Build history of the part. All positions in model axes, mm. A direction names the side the tool comes from. Give positions to 0.01 mm unless a question says otherwise; leave off trailing zeros. Write each loop counter-clockwise with the first axis right and the second up, starting at its lowest first coordinate (ties: lowest second). Pieces come first, ordered by that corner, then holes. Notation, with made-up numbers: (16.5, 54) -> (62.5, 54) arc R18 ccw to (62.5, 67) -> close; hole circle Ø7 at (51.5, -27.5). An arc over 180 degrees is marked (long way). Put each result on its own line as item: value. Start each with the question number.
Item 1: Two-plate mould, pull along Y, no slides. Class faces 1 (the flat face through (8.9, 9.4, 400.05)), 2 (the cylindrical face through (11.721, -22.534, 432.346)), 3 (the flat face through (112, -46, 0)): pulls with the +Y half, pulls with the -Y half, needs draft (parallel to the pull), parting line crosses it, or undercut.
Item 2: Tool access for faces 4 (the flat face through (5, 12, 457.2)), 5 (the cylindrical face through (-120.533, 5.305, 24.606)): list every direction of +Z, -Z, +X, -X, +Y, -Y with a clear straight run to the whole face (end or side of a thin tool).
Item 3: Drill centre lines: line 1 along Y through (x, z) = (0, 404.5); line 2 along Y through (x, z) = (0, 445.5); line 3 along X through (y, z) = (-77.5, 64). Where is each one in solid material? Low to high.
Item 4: Slice it at A-A, the plane z = 252.5. List the corners of the cut face in (x, y).
Item 5: Flat gauge pins, fed straight in: pin 1 Ø10 at (y, z) = (93.5, 150) entering from -X; pin 2 Ø10 at (x, z) = (60.5, 155.5) entering from +Y; pin 3 Ø4 at (x, z) = (-33, 144.5) entering from +Y. Where does each tip first touch, or does it go through?
```python
from build123d import *

# Parameters (mm, degrees)
F0_R     = 127
F1_DEPTH = 406.4
F2_SIZE2 = 101.6
F2_SIZE  = 355.6
F3_T     = -6.35
F4_R     = 12.7
F5_DEPTH = 25.4
F6_R     = 25.4
F6_R_2   = 12.7
F7_DEPTH = 50.8
F8_R     = 12.7


with BuildPart() as f1:
    # F0 (on Top) → F1 (new body)
    with BuildSketch(Plane.XY):
        Circle(F0_R)
    extrude(amount=F1_DEPTH)

    # F2
    f2_edges = [f1.edges().sort_by_distance(p)[0] for p in [
        (-127, 0, 406.4),
    ]]
    f2_side = f1.faces().sort_by_distance((-127, 0, 203.2))[0]
    chamfer(f2_edges, length=F2_SIZE, length2=F2_SIZE2, reference=f2_side)

    # F3
    f3_openings = [f1.faces().sort_by_distance(p)[0] for p in [
        (0, 0, 0),
    ]]
    offset(amount=F3_T, openings=f3_openings)

    # F4 (on face) → F5 (cut)
    with BuildSketch(Plane.XY.offset(406.4)):
        Circle(F4_R)
    extrude(amount=-F5_DEPTH, mode=Mode.SUBTRACT)

    # F6 (on face) → F7 (join)
    with BuildSketch(Plane.XY.offset(406.4)):
        Circle(F6_R)
        Circle(F6_R_2, mode=Mode.SUBTRACT)
    extrude(amount=F7_DEPTH)

    # F8
    f8_edges = [f1.edges().sort_by_distance(p)[0] for p in [
        (-25.4, 0, 406.4),
    ]]
    fillet(f8_edges, radius=F8_R)


solid = f1.part
```
Values follow:
1. face 1: undercut
1. face 2: parting line crosses it
1. face 3: needs draft
2. face 4: +Z, +X, -X, +Y, -Y
2. face 5: -Z
3. line 1: -25.94 to -12.7, 12.7 to 25.94
3. line 2: -25.4 to -12.7, 12.7 to 25.4
3. line 3: -95.81 to -87.15, 87.15 to 95.81
4. outline: circle Ø138.74 at (0, 0); hole circle Ø125.53 at (0, 0)
5. pin 1: x = -44.1
5. pin 2: y = 80.07
5. pin 3: y = 95.55
